Here's how the part is built. I have some questions about the finished solid (model axes, mm). A direction names the side the tool comes from. Give positions to 0.01 mm unless a question says otherwise; leave off trailing zeros. Order: outer loops, then holes, each group sorted by start corner. A loop starts at its lowest first (then second) coordinate and runs counter-clockwise, first axis right, second up. Notation, with made-up numbers: M -26.75,53.5 L 8.25,53.5 A27 cw 8.25,81.5 Z; hole C 85,-25 d9. An arc over 180 degrees is marked long. Use one line per item in the form item = value.
from build123d import *

# Parameters (mm, degrees)
SKETCH1_W           = 101.6
SKETCH1_H           = 101.6
BOSS_EXTRUDE1_DEPTH = 8.255
SKETCH3_W           = 97.536
SKETCH3_H           = 97.536
CUT_EXTRUDE1_DEPTH  = 6.223
SKETCH4_W           = 21.321387129
SKETCH4_H           = 19.016372304
BOSS_EXTRUDE2_DEPTH = 9.525
SKETCH6_W           = 17.257387129
SKETCH6_H           = 14.952372304
CUT_EXTRUDE2_DEPTH  = 9.525


with BuildPart() as part:
    # Sketch1 → Boss-Extrude1 (new body)
    with BuildSketch(Plane.XY):
        Rectangle(SKETCH1_W, SKETCH1_H)
    extrude(amount=BOSS_EXTRUDE1_DEPTH)

    # Sketch3 → Cut-Extrude1 (cut)
    with BuildSketch(Plane.XY.offset(8.255)):
        Rectangle(SKETCH3_W, SKETCH3_H)
    extrude(amount=-CUT_EXTRUDE1_DEPTH, mode=Mode.SUBTRACT)

    # Sketch4 → Boss-Extrude2 (add)
    with BuildSketch(Plane.XY.offset(2.032)):
        with Locations((27.439306436, 28.591813848)):
            Rectangle(SKETCH4_W, SKETCH4_H)
    extrude(amount=BOSS_EXTRUDE2_DEPTH)

    # Sketch6 → Cut-Extrude2 (cut)
    with BuildSketch(Plane(origin=(0, 0, 0), x_dir=(-1, 0, 0), z_dir=(0, 0, -1))):
        with Locations((-27.439306436, 28.591813848)):
            Rectangle(SKETCH6_W, SKETCH6_H)
    extrude(amount=-CUT_EXTRUDE2_DEPTH, mode=Mode.SUBTRACT)


solid = part.part
Q1. I want a section at B-B on y = -8.5. Write out the boundary of the cut face in (x, z) (3 decimals).
Found:
outline = M -50.8,0 L 50.8,0 L 50.8,8.255 L 48.768,8.255 L 48.768,2.032 L -48.768,2.032 L -48.768,8.255 L -50.8,8.255 Z
Q2. Thinking about a two-plate mould opening in X: for faces 4 (the face through (-1, 48.768, 5)), 5 (the face through (27, 29, 11.557)), 6 (the face through (50.8, -1, 4)), 7 (the face through (-50.8, -1, 4)), which applies, +X half, -X half, draft (parallel to the pull), parting line (faces both ways), or undercut?
Found:
face_4 = undercut
face_5 = draft
face_6 = +X half
face_7 = -X half
Q3. I want a section at D-D on x = 25. Write out the boundary of the cut face in (y, z) (3 decimals).
Found:
outline = M -50.8,0 L 21.116,0 L 21.116,9.525 L 36.068,9.525 L 36.068,0 L 50.8,0 L 50.8,8.255 L 48.768,8.255 L 48.768,2.032 L 38.1,2.032 L 38.1,11.557 L 19.084,11.557 L 19.084,2.032 L -48.768,2.032 L -48.768,8.255 L -50.8,8.255 Z
Q4. I need wall thicknesses on L1, parallel to Y at x = 34, z = 4.5; L2, parallel to X at y = -31.5, z = 5. Which ranges of each line are inside material? Lowest first, please.
Found:
L1 = -50.8 to -48.77, 19.08 to 21.12, 36.07 to 38.1, 48.77 to 50.8
L2 = -50.8 to -48.77, 48.77 to 50.8
Q5. I'm going to push flat-ended pins straight in: pin 1 Ø8 at (x, y) = (-32, -13) entering from +Z; pin 2 Ø3 at (y, z) = (-25.5, 10) entering from +X; pin 3 Ø7.5 at (x, y) = (29, 31) entering from -Z (3 decimals). Where does each tip first touch, or does it pass through?
Found:
pin_1 = 2.03
pin_2 = through
pin_3 = 9.525
Q6. I want a section at A-A on z = 6.25. Write out the boundary of the cut face in (x, y).
Found:
outline = M -50.8,-50.8 L 50.8,-50.8 L 50.8,50.8 L -50.8,50.8 Z; M 16.78,19.08 L 38.1,19.08 L 38.1,38.1 L 16.78,38.1 Z; hole M -48.77,-48.77 L 48.77,-48.77 L 48.77,48.77 L -48.77,48.77 Z; hole M 18.81,21.12 L 36.07,21.12 L 36.07,36.07 L 18.81,36.07 Z
Q7. On a 3-axis mill with a long thin cutter (end or side, diameter ignored), from which of +Z, -Z, +X, -X, +Y, -Y can I reach the whole of each face in a straight line? I mean faces 1 (the face through (-1, 1, 0)), 2 (the face through (48.768, -1, 5)), 3 (the face through (28, 29, 9.525)). Say none if no direction works.
Found:
face_1 = -Z, +X, -X, +Y, -Y
face_2 = +Z
face_3 = -Z
